Geometry: final body of the model. Coordinates: model frame, mm. A direction names the side the tool comes from. Round coordinates to 2 decimals unless told otherwise and drop trailing zeros. Loops run counter-clockwise (first coordinate to the right, second up) from the corner with the lowest first, then second, coordinate; pieces in that order, holes last. Notation, with made-up numbers: M -20,57 L 18,57 A13 cw 18,70 Z; hole C -11.5,-36.5 d2. An arc over 180 degrees is marked long. Return JSON: item names as keys, results as strings.
from build123d import *

# Parameters (mm, degrees)
F1_DEPTH       = 70
F3_D           = 6.6
F3_DEPTH       = 12
F3_CBORE_D     = 11.25
F3_CBORE_DEPTH = 6
F3_TIP         = 1.9828400428
F4_R           = 7.5
F5_DEPTH       = 2
F6_R           = 3.25
F7_R           = 3.25
F8_DEPTH       = 25


with BuildPart() as f1:
    # F0 (on Front) → F1 (new body, symmetric)
    with BuildSketch(Plane.XZ):
        Polygon((0, 10), (0, 0), (70, 0), (70, 40), (60, 40), (60, 10), align=None)
    extrude(amount=F1_DEPTH, both=True)

    # F3
    with Locations(Plane.XY.offset(10)):
        with Locations((12, 50), (52, 50), (52, -50), (12, -50)):
            CounterBoreHole(F3_D / 2, F3_CBORE_D / 2, F3_CBORE_DEPTH, depth=F3_DEPTH)
            with Locations((0, 0, -(F3_DEPTH + F3_TIP / 2))):  # 118° drill point
                Cone(0, F3_D / 2, F3_TIP, mode=Mode.SUBTRACT)

    # F4 (on face) → F5 (cut)
    with BuildSketch(Plane.YZ.offset(70)):
        with Locations((-55, 20)):
            Circle(F4_R)
        with Locations((55, 20)):
            Circle(F4_R)
    extrude(amount=-F5_DEPTH, mode=Mode.SUBTRACT)

    # F6 (on face) + F7 (on face) → F8 (cut)
    with BuildSketch(Plane.YZ.offset(68)):
        with Locations((-55, 20)):
            Circle(F6_R)
    with BuildSketch(Plane.YZ.offset(68)):
        with Locations((55, 20)):
            Circle(F7_R)
    extrude(amount=-F8_DEPTH, mode=Mode.SUBTRACT)


solid = f1.part
Q1. Pull-direction query (X, two-part tool) for faces 6 (the flat face through (65, -1, 40)), 7 (the cylindrical face through (11.268, -44.423, 7.042)), 8 (the flat face through (70, -1, 20)); classes: pulls with the +X half, pulls with the -X half, needs draft (parallel to the pull), parting line crosses it, or undercut.
Determined:
{"face 6": "needs draft", "face 7": "undercut", "face 8": "pulls with the +X half"}
Q2. Reachability of faces 1 (the flat face through (30, -1, 10)), 2 (the flat face through (35, -1, 0)), 3 (the cylindrical face through (54.43, -47.77, 1.97)), 4 (the cylindrical face through (55.024, 54.743, 7.042)), 5 (the cylindrical face through (69.014, -55.976, 27.436)) from +Z, -Z, +X, -X, +Y, -Y: full face, straight path, thin tool, end or side. Return the list, or none.
Determined:
{"face 1": "+Z, -X, +Y, -Y", "face 2": "-Z, +X, -X, +Y, -Y", "face 3": "+Z, -Z", "face 4": "+Z", "face 5": "+X"}
Q3. Section query D-D (y = 50). Output: boundary loops of the cut face in (x, z) (3 decimals).
Determined:
{"outline": "M 0,0 L 8.7,0 L 8.7,4 L 6.375,4 L 6.375,10 L 0,10 Z; M 15.3,0 L 48.7,0 L 48.7,4 L 46.375,4 L 46.375,10 L 17.625,10 L 17.625,4 L 15.3,4 Z; M 55.3,0 L 70,0 L 70,14.41 L 68,14.41 L 68,25.59 L 70,25.59 L 70,40 L 60,40 L 60,10 L 57.625,10 L 57.625,4 L 55.3,4 Z"}
Q4. Material intervals for L1, parallel to Y at x = 12, z = 5 (3 decimals); L2, parallel to Z at x = 64.25, y = -55; L3, parallel to Z at x = 69.1, y = -55, sorted ascending.
Determined:
{"L1": "y = -70 to -55.625, -44.375 to 44.375, 55.625 to 70", "L2": "z = 0 to 16.75, 23.25 to 40", "L3": "z = 0 to 12.5, 27.5 to 40"}
Q5. Pin query (flat end, axial travel): pin 1 (9 mm diameter, centred on x = 14, y = -50.5, fed in from +Z); pin 2 (7.5 mm diameter, centred on y = 58, z = 16.5, fed in from +X); pin 3 (1 mm diameter, centred on y = -14, z = 15.5, fed in from -X); pin 4 (10.5 mm diameter, centred on x = 12, y = -50, fed in from +Z). Return the tip coordinate at first contact, or that it passes through.
Determined:
{"pin 1": "stops at z = 10", "pin 2": "stops at x = 70", "pin 3": "stops at x = 60", "pin 4": "stops at z = 4"}
Q6. Section query B-B (x = 52). Output: boundary loops of the cut face in (y, z) (3 decimals), plus the area to 3 significant figures.
Determined:
{"outline": "M -70,0 L -53.3,0 L -53.3,4 L -55.625,4 L -55.625,10 L -70,10 Z; M -46.7,0 L 46.7,0 L 46.7,4 L 44.375,4 L 44.375,10 L -44.375,10 L -44.375,4 L -46.7,4 Z; M 53.3,0 L 70,0 L 70,10 L 55.625,10 L 55.625,4 L 53.3,4 Z", "area": "1,210 mm^2"}
Q7. Section query C-C (y = 16.5). Output: boundary loops of the cut face in (x, z), plus the area to 3 significant figures.
Determined:
{"outline": "M 0,0 L 70,0 L 70,40 L 60,40 L 60,10 L 0,10 Z", "area": "1,000 mm^2"}
Q8. Section query A-A (z = 20). Output: boundary loops of the cut face in (x, y).
Determined:
{"outline": "M 60,-70 L 70,-70 L 70,-62.5 L 68,-62.5 L 68,-58.25 L 60,-58.25 Z; M 60,-51.75 L 68,-51.75 L 68,-47.5 L 70,-47.5 L 70,47.5 L 68,47.5 L 68,51.75 L 60,51.75 Z; M 60,58.25 L 68,58.25 L 68,62.5 L 70,62.5 L 70,70 L 60,70 Z"}
